```python
from build123d import *

# Parameters (mm, degrees)
EXTRUDE3_DEPTH = 6.35


with BuildPart() as part:
    # Sketch12 → Extrude3 (new body)
    with BuildSketch(Plane(origin=(0, 0, 0), x_dir=(1, 0, 0), z_dir=(0, 1, 0))):
        with BuildLine():
            Line((47.659255792, 0), (-47.659255792, 0))
            ThreePointArc((-47.659255792, 0), (-64.107574089, 29.295195073), (-70.144576115, 62.345312104))
            ThreePointArc((-70.144576115, 62.345312104), (-64.669164862, 76.002515657), (-51.096777519, 81.684912961))
            Line((-51.096777519, 81.684912961), (51.096777519, 81.684912961))
            ThreePointArc((51.096777519, 81.684912961), (64.669164862, 76.002515657), (70.144576115, 62.345312104))
            ThreePointArc((70.144576115, 62.345312104), (64.107574089, 29.295195073), (47.659255792, 0))
        make_face()
    extrude(amount=-EXTRUDE3_DEPTH)


solid = part.part
```
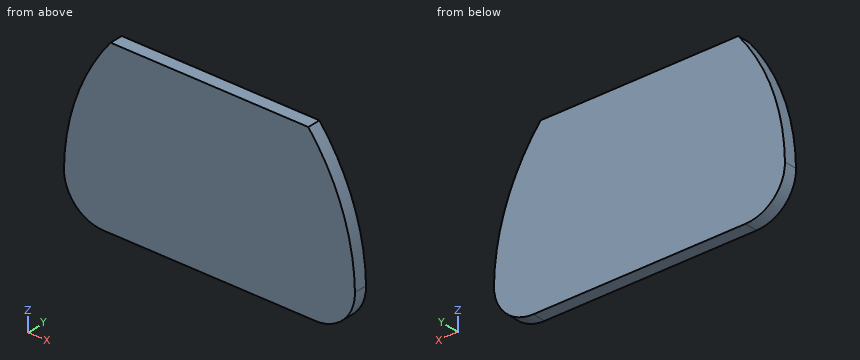
Work out the finished part from the listing and answer in its coordinate system (mm). Give positions to 0.01 mm unless a question says otherwise; leave off trailing zeros. Write each loop counter-clockwise with the first axis right and the second up, starting at its lowest first coordinate (ties: lowest second). Pieces come first, ordered by that corner, then holes. Notation, with made-up numbers: (14, 70.5) -> (39, 70.5) arc R26 cw to (39, 99.5) -> close; hole circle Ø7 at (-23.75, 46). An arc over 180 degrees is marked (long way). Write item = value, one per line.
Q1. Section C-C on x = 52.5 is taken. Determine the outline of the cut face in (y, z), and give its area (3 significant figures).
Computed values:
outline = (-6.35, -81.63) -> (0, -81.63) -> (0, -6.54) -> (-6.35, -6.54) -> close
area = 477 mm^2
Q2. Consider line 1 along X through (y, z) = (-2, -74); line 2 along Z through (x, y) = (51, -0.75); line 3 along X through (y, z) = (-6, -39). Determine where each line is inside the solid, lowest interval first.
Computed values:
line_1 = -66.39 to 66.39
line_2 = -81.68 to -4.39
line_3 = -67.07 to 67.07
Q3. Section A-A on y = -2 is taken. Determine the outline of the cut face in (x, z), and give its area (3 significant figures).
Computed values:
outline = (-70.14, -62.35) arc R19.05 ccw to (-51.1, -81.68) -> (51.1, -81.68) arc R19.05 ccw to (70.14, -62.35) arc R101.99 ccw to (47.66, 0) -> (-47.66, 0) arc R101.99 ccw to start
area = 10,400 mm^2
Q4. Section B-B on z = -33.5 is taken. Determine the outline of the cut face in (x, y), and give its area (3 significant figures).
Computed values:
outline = (-65.52, -6.35) -> (65.52, -6.35) -> (65.52, 0) -> (-65.52, 0) -> close
area = 832 mm^2
Q5. Flat-ended cylindrical pins translate along their axes: pin 1 Ø3 at (y, z) = (-4, -66) entering from -X; pin 2 Ø4 at (x, z) = (16.5, -19) entering from +Y. Find the tip coordinate at first contact, or state that the pin passes through.
Computed values:
pin_1 = -70.06
pin_2 = 0
